Read the model definition and answer for the solid it produces. Units are mm, in the model's axes. A direction names the side the tool comes from. Give positions to 0.01 mm unless a question says otherwise; leave off trailing zeros. Order: outer loops, then holes, each group sorted by start corner. A loop starts at its lowest first (then second) coordinate and runs counter-clockwise, first axis right, second up.
```python
from build123d import *

# Parameters (mm, degrees)
MODEL_R         = 2.761626555
MODEL_R_2       = 1.866571664
MODEL_R_3       = 1.313234148
MODEL_R_4       = 2.116722719
MODEL_R_5       = 1.509742993
EXTRUDE_1_DEPTH = 1.5


with BuildPart() as part:
    # Model → 凸台-拉伸1 (new body)
    with BuildSketch(Plane.XY):
        Polygon((244.059423642, -194.252615776), (166.526919178, -199.674216635), (166.526919178, -195.252615776), (164.526919178, -195.252615776), (164.526919178, -190.252615776), (166.526919178, -190.252615776), (166.526919178, -185.831017216), (244.059416516, -191.252615776), (244.059417704, -191.752615776), (238.059420079, -191.752615776), (238.059420079, -192.752615776), (238.059420079, -193.752615776), (244.059422454, -193.752615776), align=None)
        with Locations((177.162967315, -192.752615776)):
            Circle(MODEL_R, mode=Mode.SUBTRACT)
        with Locations((197.250125118, -192.752615776)):
            Circle(MODEL_R_2, mode=Mode.SUBTRACT)
        with Locations((214.974129703, -192.752615776)):
            Circle(MODEL_R_3, mode=Mode.SUBTRACT)
        with Locations((186.829055112, -192.752615776)):
            Circle(MODEL_R_4, mode=Mode.SUBTRACT)
        with Locations((206.302954902, -192.752615776)):
            Circle(MODEL_R_5, mode=Mode.SUBTRACT)
    extrude(amount=EXTRUDE_1_DEPTH)


solid = part.part
```
1) The part is cut by section B-B on z = 0.65. Determine the outline of the cut face in (x, y), and give its area (3 significant figures).
Final values:
outline: (164.53, -195.25) - (166.53, -195.25) - (166.53, -199.67) - (244.06, -194.25) - (244.06, -193.75) - (238.06, -193.75) - (238.06, -191.75) - (244.06, -191.75) - (244.06, -191.25) - (166.53, -185.83) - (166.53, -190.25) - (164.53, -190.25) - close; hole circle Ø5.52 at (177.16, -192.75); hole circle Ø4.23 at (186.83, -192.75); hole circle Ø3.73 at (197.25, -192.75); hole circle Ø3.02 at (206.3, -192.75); hole circle Ø2.63 at (214.97, -192.75)
area: 589 mm2
2) For a pull along Y with two mould halves and no side action, classify faces 4 (the face through (241, -191.753, 1)), 5 (the face through (204.75, -188.504, 0.74)), 6 (the face through (166.527, -188, 1)) as released by +Y, released by -Y, zero draft, split by the parting line, or undercut.
Final values:
face 4: undercut
face 5: released by +Y
face 6: zero draft
3) A tool of negligible diameter and unlimited length cuts with its end or side. For faces 1 (the face through (166, -190.253, 1)), 2 (the face through (166, -195.253, 1)), 3 (the face through (238.059, -193, 1)), from which of +Z, -Z, +X, -X, +Y, -Y can it reach the whole face along a straight path? Write none if from no direction.
Final values:
face 1: +Z, -Z, -X, +Y
face 2: +Z, -Z, -X, -Y
face 3: +Z, -Z, +X
4) The part is cut by section C-C on x = 217.5. Determine the outline of the cut face in (y, z).
Final values:
outline: (-196.11, 0) - (-189.4, 0) - (-189.4, 1.5) - (-196.11, 1.5) - close
5) The part is cut by section D-D on y = -187.5. Determine the outline of the cut face in (x, z), and give its area (3 significant figures).
Final values:
outline: (166.53, 0) - (190.39, 0) - (190.39, 1.5) - (166.53, 1.5) - close
area: 35.8 mm2
6) Consider L1, parallel to X at y = -192.75, z = 0.65; L2, parallel to Y at x = 239.5, z = 0.65; L3, parallel to Y at x = 178, z = 0.1. Determine where each line is inside the solid, lowest interval first.
Final values:
L1: x = 164.53 to 174.4, 179.92 to 184.71, 188.95 to 195.38, 199.12 to 204.79, 207.81 to 213.66, 216.29 to 238.06
L2: y = -194.57 to -193.75, -191.75 to -190.93
L3: y = -198.87 to -195.38, -190.12 to -186.63
7) Given pin 1 (3.5 mm diameter, centred on x = 214.97, y = -192.75, fed in from -Z); pin 2 (0.8 mm diameter, centred on y = -193, z = 0.5, fed in from +X); pin 3 (1.8 mm diameter, centred on x = 206.3, y = -192.75, fed in from +Z); pin 4 (0.8 mm diameter, centred on y = -197.5, z = 1, fed in from -X), each flat-ended and moving along its own axis, determine where each tip first touches the part or whether it passes through.
Final values:
pin 1: stops at z = 0
pin 2: stops at x = 238.06
pin 3: passes through
pin 4: stops at x = 166.53
8) The part is cut by section A-A on x = 175.5. Determine the outline of the cut face in (y, z).
Final values:
outline: (-199.05, 0) - (-194.96, 0) - (-194.96, 1.5) - (-199.05, 1.5) - close; (-190.55, 0) - (-186.46, 0) - (-186.46, 1.5) - (-190.55, 1.5) - close
